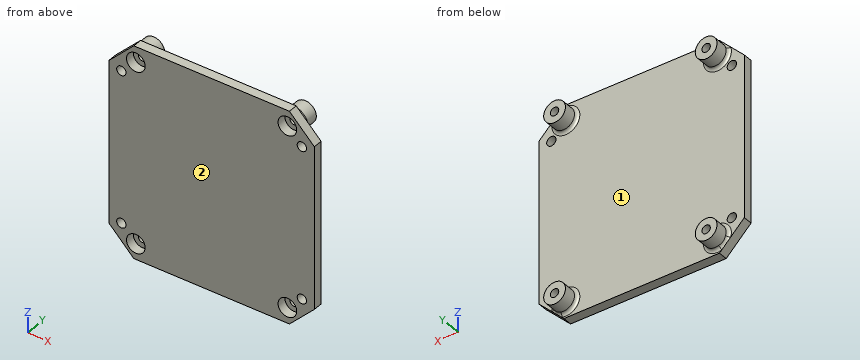
from build123d import *

# Parameters (mm, degrees)
SKETCH_1_W      = 66
SKETCH_1_H      = 68
SKETCH_1_R      = 1.5
SKETCH_1_R_2    = 3
EXTRUDE_1_DEPTH = 3
SKETCH_2_R      = 3.5
SKETCH_2_R_2    = 1.35
EXTRUDE_2_DEPTH = 5
CHAMFER_1_SIZE  = 8
FILLET_2_R      = 1


with BuildPart() as part:
    # 草图1 → 凸台-拉伸1 (new body)
    with BuildSketch(Plane(origin=(0, 0, 0), x_dir=(1, 0, 0), z_dir=(0, 1, 0))):
        Rectangle(SKETCH_1_W, SKETCH_1_H)
        with Locations(Location((-29, 24.35, 0), (0, 0, 270))):
            Circle(SKETCH_1_R, mode=Mode.SUBTRACT)
        with Locations(Location((29, 24.35, 0), (0, 0, 270))):
            Circle(SKETCH_1_R, mode=Mode.SUBTRACT)
        with Locations(Location((29, -24.35, 0), (0, 0, 270))):
            Circle(SKETCH_1_R, mode=Mode.SUBTRACT)
        with Locations(Location((-29, -24.35, 0), (0, 0, 270))):
            Circle(SKETCH_1_R, mode=Mode.SUBTRACT)
        with Locations(Location((-24.35, 29, 0), (0, 0, 270))):
            Circle(SKETCH_1_R_2, mode=Mode.SUBTRACT)
        with Locations(Location((24.35, 29, 0), (0, 0, 270))):
            Circle(SKETCH_1_R_2, mode=Mode.SUBTRACT)
        with Locations(Location((-24.35, -29, 0), (0, 0, 270))):
            Circle(SKETCH_1_R_2, mode=Mode.SUBTRACT)
        with Locations(Location((24.35, -29, 0), (0, 0, 270))):
            Circle(SKETCH_1_R_2, mode=Mode.SUBTRACT)
    extrude(amount=EXTRUDE_1_DEPTH)

    # 草图2 → 凸台-拉伸2 (add)
    # profile 1 of 4: a face of its own
    with BuildSketch(Plane(origin=(0, 3, 0), x_dir=(1, 0, 0), z_dir=(0, 1, 0))):
        with Locations(Location((-24.35, 29, 0), (0, 0, 270))):
            Circle(SKETCH_2_R)
        with Locations(Location((-24.35, 29, 0), (0, 0, 270))):
            Circle(SKETCH_2_R_2, mode=Mode.SUBTRACT)
    # profile 2 of 4: a face of its own
    with BuildSketch(Plane(origin=(0, 3, 0), x_dir=(1, 0, 0), z_dir=(0, 1, 0))):
        with Locations(Location((24.35, 29, 0), (0, 0, 90))):
            Circle(SKETCH_2_R)
        with Locations(Location((24.35, 29, 0), (0, 0, 90))):
            Circle(SKETCH_2_R_2, mode=Mode.SUBTRACT)
    # profile 3 of 4: a face of its own
    with BuildSketch(Plane(origin=(0, 3, 0), x_dir=(1, 0, 0), z_dir=(0, 1, 0))):
        with Locations(Location((24.35, -29, 0), (0, 0, 270))):
            Circle(SKETCH_2_R)
        with Locations(Location((24.35, -29, 0), (0, 0, 270))):
            Circle(SKETCH_2_R_2, mode=Mode.SUBTRACT)
    # profile 4 of 4: a face of its own
    with BuildSketch(Plane(origin=(0, 3, 0), x_dir=(1, 0, 0), z_dir=(0, 1, 0))):
        with Locations(Location((-24.35, -29, 0), (0, 0, 90))):
            Circle(SKETCH_2_R)
        with Locations(Location((-24.35, -29, 0), (0, 0, 90))):
            Circle(SKETCH_2_R_2, mode=Mode.SUBTRACT)
    extrude(amount=EXTRUDE_2_DEPTH)

    # 倒角1
    chamfer_1_edges = [part.edges().sort_by_distance(p)[0] for p in [
        (-33, 1.5, -34),
        (33, 1.5, -34),
        (33, 1.5, 34),
        (-33, 1.5, 34),
    ]]
    chamfer(chamfer_1_edges, length=CHAMFER_1_SIZE)

    # 圆角2
    fillet_2_edges = [part.edges().sort_by_distance(p)[0] for p in [
        (-24.35, 3, 32.5),
        (24.35, 3, 25.5),
        (24.35, 3, -25.5),
        (-24.35, 3, -32.5),
    ]]
    fillet(fillet_2_edges, radius=FILLET_2_R)


solid = part.part
Work out the finished part from the listing and answer in its coordinate system (mm). Face numbers are marked on the shaded views. Round coordinates to 2 decimals unless told otherwise and drop trailing zeros. Order: outer loops, then holes, each group sorted by start corner. A loop starts at its lowest first (then second) coordinate and runs counter-clockwise, first axis right, second up. Notation, with made-up numbers: M -9.75,5 L 16.25,5 A9 ccw 16.25,22 Z; hole C 73.5,12 d4. An arc over 180 degrees is marked long. One line per item, written item: value.
Q1. Find section D-D on x = 15. Write down the section's boundary in (y, z), then the cut area to 3 significant figures.
Derived:
outline: M 0,-34 L 3,-34 L 3,34 L 0,34 Z
area: 204 mm²
Q2. Flat-ended cylindrical pins translate along their axes: pin 1 (3 mm diameter, centred on x = 25, z = 29.5, fed in from -Y); pin 2 (20 mm diameter, centred on x = 13, z = 8.5, fed in from +Y). Find the tip coordinate at first contact, or state that the pin passes through.
Derived:
pin 1: y = 3
pin 2: y = 3
Q3. Find section B-B on z = -29. Give the number of separate pieces and of enclosed holes in the cut face, then the cut area to 3 significant figures.
Derived:
separate pieces: 3
enclosed holes: 0
area: 188 mm²
Q4. Straight lines are drawn through the part: line 1 (X direction, y = 1.45, z = 24.35); line 2 (Z direction, x = -30, y = 1.75); line 3 (X direction, y = 1.95, z = 29). For each, find the intervals that lie inside material, in ascending order.
Derived:
line 1: -33 to -30.5, -27.5 to 27.5, 30.5 to 33
line 2: -29 to -25.47, -23.23 to 23.23, 25.47 to 29
line 3: -30 to -27.35, -21.35 to 21.35, 27.35 to 30
Q5. Find section A-A on y = 6.25. Write down the section's boundary in (x, z), then the cut area to 3 significant figures.
Derived:
outline: C -24.35,-29 d7; C -24.35,29 d7; C 24.35,-29 d7; C 24.35,29 d7; hole C -24.35,-29 d2.7; hole C -24.35,29 d2.7; hole C 24.35,-29 d2.7; hole C 24.35,29 d2.7
area: 131 mm²
Q6. Determine the mould class of the marked faces 1 and 2 for opening direction X: released by +X, released by -X, zero draft, split by the parting line, or undercut.
Derived:
face 1: undercut
face 2: zero draft
Q7. Find section C-C on z = -16. Write down the section's boundary in (x, y), then the cut area to 3 significant figures.
Derived:
outline: M -33,0 L 33,0 L 33,3 L -33,3 Z
area: 198 mm²
